from build123d import *

# Parameters (mm, degrees)
SKETCH1_R                   = 4
BOSS_EXTRUDE1_DEPTH         = 5
FILLET1_R                   = 2
M4_TAPPED_HOLE1_D           = 3.3
M4_TAPPED_HOLE1_CSINK_D     = 4.05
M4_TAPPED_HOLE1_CSINK_ANGLE = 90


with BuildPart() as part:
    # Sketch1 → Boss-Extrude1 (new, symmetric)
    with BuildSketch(Plane.XY):
        Polygon((-35, 0), (35, 0), (35, 9), (30.8, 9), (26.8, 13), (16.8, 13), (12, 4), (-12, 4), (-16.8, 13), (-26.8, 13), (-30.8, 9), (-35, 9), align=None)
        with Locations((22, 7)):
            Circle(SKETCH1_R, mode=Mode.SUBTRACT)
        with Locations(Location((-22, 7, 0), (0, 0, 180))):
            Circle(SKETCH1_R, mode=Mode.SUBTRACT)
    extrude(amount=BOSS_EXTRUDE1_DEPTH, both=True)

    # Fillet1
    fillet1_edges = [part.edges().sort_by_distance(p)[0] for p in [
        (-30.8, 9, 0),
        (-26.8, 13, 0),
        (-16.8, 13, 0),
        (-12, 4, 0),
        (12, 4, 0),
        (16.8, 13, 0),
        (26.8, 13, 0),
        (30.8, 9, 0),
    ]]
    fillet(fillet1_edges, radius=FILLET1_R)

    # M4 Tapped Hole1 (through all)
    with Locations(Plane(origin=(0, 0, 0), x_dir=(-1, 0, 0), z_dir=(0, -1, 0))):
        with Locations((-30, 0), (30, 0)):
            CounterSinkHole(M4_TAPPED_HOLE1_D / 2, M4_TAPPED_HOLE1_CSINK_D / 2, counter_sink_angle=M4_TAPPED_HOLE1_CSINK_ANGLE)


solid = part.part
Source: CAD feature listing. Evaluate the final solid. Frame: model axes, mm. A direction names the side the tool comes from. Give positions to 0.01 mm unless a question says otherwise; leave off trailing zeros. Write each loop counter-clockwise with the first axis right and the second up, starting at its lowest first coordinate (ties: lowest second). Pieces come first, ordered by that corner, then holes. Notation, with made-up numbers: (-6.5, 56) -> (50.5, 56) arc R26 cw to (50.5, 83) -> close; hole circle Ø3 at (45.5, 8.5). An arc over 180 degrees is marked (long way). Return JSON: item names as keys, results as strings. Group by question number.
1. Material intervals for line 1 (Y direction, x = -22, z = -2.5); line 2 (X direction, y = 4.25, z = -3.75); line 3 (Z direction, x = -30, y = 7), sorted ascending. Write a range as from..to.
2. Section B-B, the plane z = 2.75. Output: boundary loops of the cut face in (x, y).
3. Section D-D, the plane x = -3.5. Output: boundary loops of the cut face in (y, z).
4. Mould query, pull axis Y, two halves, no side actions, for faces 1 (the face through (-18.8, 9.4, -0.1)), 2 (the face through (28.35, 4.76, -0.07)), 3 (the face through (22, 13, 0)), 4 (the face through (18, 7, 0)). Classes: +Y half, -Y half, draft (parallel to the pull), parting line (faces both ways), or undercut.
5. Section C-C, the plane x = -22. Output: boundary loops of the cut face in (y, z), then the cut area to 3 significant figures.
6. Pin query (flat end, axial travel): pin 1 Ø4.5 at (x, z) = (30, 0) entering from +Y; pin 2 Ø1.5 at (x, z) = (-26, 1.5) entering from -Y; pin 3 Ø3.5 at (x, z) = (-32.5, 0) entering from +Y; pin 4 Ø2.5 at (x, z) = (33.5, 0.5) entering from +Y. Return the tip coordinate at first contact, or that it passes through.
7. Section A-A, the plane y = 7. Output: boundary loops of the cut face in (x, z).
8. Access query for faces 5 (the face through (-33, 9, 0)), 6 (the face through (16.96, 12.71, 0.07)), 7 (the face through (0, 0, 0)). Directions: +Z, -Z, +X, -X, +Y, -Y. A direction counts if a zero-diameter tool reaches every point of the face in a straight line with its end or side. Return the directions, or none.
Determined:
{
 "1": {"line 1": "y = 0..3, 11..13", "line 2": "x = -35..-24.9, -19.1..-11.77, 11.77..19.1, 24.9..35", "line 3": "z = -5..-1.65, 1.65..5"},
 "2": {"outline": "(-35, 0) -> (35, 0) -> (35, 9) -> (31.63, 9) arc R2 cw to (30.21, 9.59) -> (27.39, 12.41) arc R2 ccw to (25.97, 13) -> (18, 13) arc R2 ccw to (16.24, 11.94) -> (12.56, 5.06) arc R2 cw to (10.8, 4) -> (-10.8, 4) arc R2 cw to (-12.56, 5.06) -> (-16.24, 11.94) arc R2 ccw to (-18, 13) -> (-25.97, 13) arc R2 ccw to (-27.39, 12.41) -> (-30.21, 9.59) arc R2 cw to (-31.63, 9) -> (-35, 9) -> close; hole circle Ø8 at (-22, 7); hole circle Ø8 at (22, 7)"},
 "3": {"outline": "(0, -5) -> (4, -5) -> (4, 5) -> (0, 5) -> close"},
 "4": {"face 1": "undercut", "face 2": "draft", "face 3": "+Y half", "face 4": "undercut"},
 "5": {"outline": "(0, -5) -> (3, -5) -> (3, 5) -> (0, 5) -> close; (11, -5) -> (13, -5) -> (13, 5) -> (11, 5) -> close", "area": "50.0 mm2"},
 "6": {"pin 1": "stops at y = 12.05", "pin 2": "stops at y = 0", "pin 3": "stops at y = 9.05", "pin 4": "stops at y = 9"},
 "7": {"outline": "(-35, -5) -> (-26, -5) -> (-26, 5) -> (-35, 5) -> close; (-18, -5) -> (-13.6, -5) -> (-13.6, 5) -> (-18, 5) -> close; (13.6, -5) -> (18, -5) -> (18, 5) -> (13.6, 5) -> close; (26, -5) -> (35, -5) -> (35, 5) -> (26, 5) -> close; hole circle Ø3.3 at (-30, 0); hole circle Ø3.3 at (30, 0)"},
 "8": {"face 5": "+Z, -Z, -X, +Y", "face 6": "+Z, -Z, +Y", "face 7": "+Z, -Z, +X, -X, -Y"}
}
